Geometry check sheet. Reference: the model listing, model coordinates, mm. Face numbers are marked on the shaded views. A direction names the side the tool comes from. Give positions to 0.01 mm unless a question says otherwise; leave off trailing zeros. Write each loop counter-clockwise with the first axis right and the second up, starting at its lowest first coordinate (ties: lowest second). Pieces come first, ordered by that corner, then holes.
(1) Thickness scan on line 1 along Z through (x, y) = (16, 0.5); line 2 along Z through (x, y) = (12, 2.6); line 3 along Z through (x, y) = (-22, 1.65). Record the ranges inside material, lowest first.
(2) Cross-section at A-A (y = 0.9). Count the separate pieces of the cut face and the enclosed holes in it, and give its area (3 significant figures).
(3) Tool access check on the marked faces 3 and 4. Record the directions out of +Z, -Z, +X, -X, +Y, -Y that give a thin tool (end or side, any length) a straight path to the whole face; none if there is none.
(4) Mould release check, pull along X, two halves, no side actions. Record for the marked faces 1 and 2: +X half, -X half, draft (parallel to the pull), parting line (faces both ways), or undercut.
(5) Cross-section at C-C (x = -4). Record the boundary of the cut face in (y, z).
(6) Cross-section at D-D (x = -15.5). Record the boundary of the cut face in (y, z) (3 decimals), and give its area (3 significant figures).
(7) Cross-section at B-B (x = 24). Record the boundary of the cut face in (y, z), and give its area (3 significant figures).
(8) Depth check by flat-ended pin: P1, Ø1.6, axis at x = 12, z = 4, coming from the -Y side; P2, Ø1.6, axis at x = -20, z = 3.5, coming from the -Y side; P3, Ø4.5, axis at x = -16, z = 0, coming from the +Y side. Enter the tip coordinate at first touch or a pass-through.
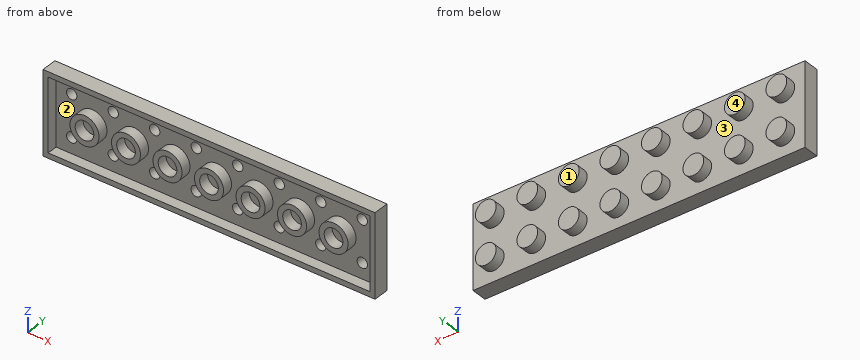
```python
from build123d import *

# Parameters (mm, degrees)
SKETCH1_W           = 64
SKETCH1_H           = 16
BOSS_EXTRUDE1_DEPTH = 3
SKETCH2_R           = 2
BOSS_EXTRUDE2_DEPTH = 2
SHELL1_T            = -1
SKETCH3_R           = 2.8
SKETCH3_R_2         = 1.8
BOSS_EXTRUDE3_DEPTH = 2
LPATTERN1_COUNT     = 7
LPATTERN1_PITCH     = 8


with BuildPart() as part:
    # Sketch1 → Boss-Extrude1 (new body)
    with BuildSketch(Plane(origin=(0, 0, 0), x_dir=(1, 0, 0), z_dir=(0, 1, 0))):
        Rectangle(SKETCH1_W, SKETCH1_H)
    extrude(amount=BOSS_EXTRUDE1_DEPTH)

    # Sketch2 → Boss-Extrude2 (add)
    with BuildSketch(Plane(origin=(0, 3, 0), x_dir=(1, 0, 0), z_dir=(0, 1, 0))):
        with Locations((-28, 4)):
            Circle(SKETCH2_R)
        with Locations((-20, 4)):
            Circle(SKETCH2_R)
        with Locations((-12, 4)):
            Circle(SKETCH2_R)
        with Locations((-4, 4)):
            Circle(SKETCH2_R)
        with Locations((4, 4)):
            Circle(SKETCH2_R)
        with Locations((12, 4)):
            Circle(SKETCH2_R)
        with Locations((20, 4)):
            Circle(SKETCH2_R)
        with Locations((28, 4)):
            Circle(SKETCH2_R)
        with Locations((-20, -4)):
            Circle(SKETCH2_R)
        with Locations((-12, -4)):
            Circle(SKETCH2_R)
        with Locations((-4, -4)):
            Circle(SKETCH2_R)
        with Locations((4, -4)):
            Circle(SKETCH2_R)
        with Locations((12, -4)):
            Circle(SKETCH2_R)
        with Locations((20, -4)):
            Circle(SKETCH2_R)
        with Locations((28, -4)):
            Circle(SKETCH2_R)
        with Locations((-28, -4)):
            Circle(SKETCH2_R)
    extrude(amount=BOSS_EXTRUDE2_DEPTH)

    # Shell1
    shell1_openings = [part.faces().sort_by_distance(p)[0] for p in [
        (0, 0, 0),
    ]]
    offset(amount=SHELL1_T, openings=shell1_openings, kind=Kind.INTERSECTION)

    # Sketch3 → Boss-Extrude3 (add)
    with BuildSketch(Plane.XZ.offset(-2)):
        with Locations((-24, 0)):
            Circle(SKETCH3_R)
        with Locations((-24, 0)):
            Circle(SKETCH3_R_2, mode=Mode.SUBTRACT)
    boss_extrude3 = extrude(amount=BOSS_EXTRUDE3_DEPTH)

    # LPattern1: Boss-Extrude3 ×7
    with Locations(*[(i * LPATTERN1_PITCH, 0, 0) for i in range(1, LPATTERN1_COUNT)]):
        add(boss_extrude3)


solid = part.part
```
Reply:
1. line 1: z = -8 to -7, -2.8 to -1.8, 1.8 to 2.8, 7 to 8
1. line 2: z = -8 to -5, -3 to 3, 5 to 8
1. line 3: z = -8 to -7, -1.96 to 1.96, 7 to 8
2. separate pieces: 8
2. enclosed holes: 8
2. area: 257 mm2
3. face 3: +Y
3. face 4: +Z, -Z, +X, -X, +Y
4. face 1: draft
4. face 2: undercut
5. outline: (0, -8) - (3, -8) - (3, -6) - (5, -6) - (5, -2) - (3, -2) - (3, 2) - (5, 2) - (5, 6) - (3, 6) - (3, 8) - (0, 8) - (0, 7) - (2, 7) - (2, 5) - (4, 5) - (4, 3) - (2, 3) - (2, -3) - (4, -3) - (4, -5) - (2, -5) - (2, -7) - (0, -7) - close
6. outline: (0, -8) - (3, -8) - (3, 8) - (0, 8) - (0, 7) - (2, 7) - (2, 2.755) - (0, 2.755) - (0, 1.729) - (2, 1.729) - (2, -1.729) - (0, -1.729) - (0, -2.755) - (2, -2.755) - (2, -7) - (0, -7) - close
6. area: 24.1 mm2
7. outline: (0, -8) - (3, -8) - (3, 8) - (0, 8) - (0, 7) - (2, 7) - (2, 2.8) - (0, 2.8) - (0, 1.8) - (2, 1.8) - (2, -1.8) - (0, -1.8) - (0, -2.8) - (2, -2.8) - (2, -7) - (0, -7) - close
7. area: 24.0 mm2
8. P1: stops at y = 4
8. P2: stops at y = 2
8. P3: stops at y = 3
